The listing builds one solid part. Answer for the finished solid, in the listing's coordinates (mm). A direction names the side the tool comes from. Give positions to 0.01 mm unless a question says otherwise; leave off trailing zeros. Write each loop counter-clockwise with the first axis right and the second up, starting at its lowest first coordinate (ties: lowest second). Pieces come first, ordered by that corner, then holes. Notation, with made-up numbers: (-22, -20.75) - (-2, -20.75) arc R36 ccw to (-2, 18.25) - close; hole circle Ø3 at (-19, 71). An arc over 180 degrees is marked (long way). Answer in a Markdown table with one row per item. Add a question column.
from build123d import *

# Parameters (mm, degrees)
PAD043_DEPTH    = 15
POCKET057_DEPTH = 13
SKETCH118_R     = 1.65
SKETCH118_R_2   = 1.7
SKETCH118_R_3   = 20
POCKET058_DEPTH = 15
POCKET059_DEPTH = 5


with BuildPart() as part:
    # Sketch116 → Pad043 (new body)
    with BuildSketch(Plane.YZ):
        with BuildLine():
            Line((27.5, -9.253658), (27.5, -51.25))
            Line((27.5, -51.25), (-27.5, -51.25))
            Line((-27.5, -51.25), (-27.5, -9.253658))
            ThreePointArc((-20.340323, 1.39583), (-25.543681, -2.837417), (-27.5, -9.253658))
            ThreePointArc((-20.340323, 1.39583), (-18.530459, 2.868264), (-17.85, 5.1))
            ThreePointArc((-12.15, 5.1), (-15, 7.95), (-17.85, 5.1))
            ThreePointArc((-12.15, 5.1), (-11.315254, 3.084746), (-9.3, 2.25))
            Line((-9.3, 2.25), (9.3, 2.25))
            ThreePointArc((9.3, 2.25), (11.315254, 3.084746), (12.15, 5.1))
            ThreePointArc((17.85, 5.1), (15, 7.95), (12.15, 5.1))
            ThreePointArc((17.85, 5.1), (18.530459, 2.868264), (20.340323, 1.39583))
            ThreePointArc((27.5, -9.253658), (25.543681, -2.837417), (20.340323, 1.39583))
        make_face()
    extrude(amount=-PAD043_DEPTH)

    # Sketch117 (on Face14 of Pad043) → Pocket057 (cut)
    with BuildSketch(Plane(origin=(-15, 0, 0), x_dir=(0, -1, 0), z_dir=(-1, 0, 0))):
        with BuildLine():
            Line((-26, -9.253658), (-26, -51.25))
            Line((-26, -51.25), (26, -51.25))
            Line((26, -51.25), (26, -9.253658))
            ThreePointArc((26, -9.253658), (23.071068, -2.18259), (16, 0.746342))
            Line((-16, 0.746342), (16, 0.746342))
            ThreePointArc((-16, 0.746342), (-23.071068, -2.18259), (-26, -9.253658))
        make_face()
    extrude(amount=-POCKET057_DEPTH, mode=Mode.SUBTRACT)

    # Sketch118 (on Face4 of Pocket057) → Pocket058 (cut)
    with BuildSketch(Plane.YZ):
        with Locations((-15, 5.1)):
            Circle(SKETCH118_R)
        with Locations((15, 5.1)):
            Circle(SKETCH118_R)
        with Locations((22.4, -44.05)):
            Circle(SKETCH118_R_2)
        with Locations((-20.9, -5.25)):
            Circle(SKETCH118_R_2)
        with Locations((2, -26.25)):
            Circle(SKETCH118_R_3)
    extrude(amount=-POCKET058_DEPTH, mode=Mode.SUBTRACT)

    # Sketch119 (on Face11 of Pocket058) → Pocket059 (cut)
    with BuildSketch(Plane(origin=(0, -27.5, 0), x_dir=(0, 0, 1), z_dir=(0, -1, 0))):
        Polygon((-51.25, 15), (-28.815971, 15), (-38.35, 7), (-51.25, 7), align=None)
    extrude(amount=-POCKET059_DEPTH, mode=Mode.SUBTRACT)


with BuildPart() as part_1:
    # Body016 placement: moved
    add(part.part.moved(Location((32, 0, 0))))


solid = part_1.part
1. Section C-C (z = -31.5) is taken. Give the vertices of the cut face in (x, y), and give its area (3 significant figures).
2. Section B-B (x = 25.75) is taken. Give the vertices of the cut face in (y, z), and give its area (3 significant figures).
3. Section A-A (y = 2) is taken. Give the vertices of the cut face in (x, z), and give its area (3 significant figures).
4. Given pin 1 Ø4 at (y, z) = (-5, -11) entering from +X; pin 2 Ø4 at (x, y) = (26.5, 13.5) entering from -Z; pin 3 Ø8 at (x, y) = (20, 13.5) entering from -Z; pin 4 Ø1 at (x, z) = (30.5, -3) entering from -Y, each flat-ended and moving along its own axis, determine where each tip first touches the part or whether it passes through.
5. Section D-D (y = -15) is taken. Give the vertices of the cut face in (x, z), and give its area (3 significant figures).
6. A tool of negligible diameter and unlimited length cuts with its end or side. For faces 5 (the face through (20.944, -26.76, -33.516)), 6 (the face through (25, 0, 2.25)), 7 (the face through (23.41, -23.15, -2.26)), 8 (the face through (32, -18, -21)), from which of +Z, -Z, +X, -X, +Y, -Y can it reach the whole face along a straight path? Write none if from no direction.
7. Straight lines are drawn through the part: L1, parallel to Y at x = 18, z = -28.5; L2, parallel to Z at x = 31, y = 2; L3, parallel to Y at x = 26.5, z = 4.5. For each, find the intervals that lie inside material, in ascending order. Write a range as [from, to].
8. The mould has two halves that part along Z. Classify faces 1 (the face through (23, 26, -30)), 2 (the face through (31, -22.6, -5.2)), 3 (the face through (23, 0, 0.746)), 4 (the face through (24.6, 25.6, -2.92)): +Z half, -Z half, draft (parallel to the pull), parting line (faces both ways), or undercut.
Geometry check:
| question | item | result |
|---|---|---|
| 1 | outline | (17, 26) - (30, 26) - (30, 21.3) - (32, 21.3) - (32, 27.5) - (17, 27.5) - close; (19.25, -27.5) - (32, -27.5) - (32, -17.3) - (30, -17.3) - (30, -26) - (19.25, -26) - close |
| 1 | area | 68.4 mm² |
| 2 | outline | (-27.5, -51.25) - (-26, -51.25) - (-26, -9.25) arc R10 cw to (-16, 0.75) - (16, 0.75) arc R10 cw to (26, -9.25) - (26, -51.25) - (27.5, -51.25) - (27.5, -9.25) arc R11.5 ccw to (20.34, 1.4) arc R4 cw to (17.85, 5.1) arc R2.85 ccw to (12.15, 5.1) arc R2.85 cw to (9.3, 2.25) - (-9.3, 2.25) arc R2.85 cw to (-12.15, 5.1) arc R2.85 ccw to (-17.85, 5.1) arc R4 cw to (-20.34, 1.4) arc R11.5 ccw to (-27.5, -9.25) - close; hole circle Ø3.3 at (-15, 5.1); hole circle Ø3.3 at (15, 5.1) |
| 2 | area | 272 mm² |
| 3 | outline | (17, 0.75) - (30, 0.75) - (30, -6.25) - (32, -6.25) - (32, 2.25) - (17, 2.25) - close; (30, -51.25) - (32, -51.25) - (32, -46.25) - (30, -46.25) - close |
| 3 | area | 46.5 mm² |
| 4 | pin 1 | through |
| 4 | pin 2 | z = 0.75 |
| 4 | pin 3 | z = 0.63 |
| 4 | pin 4 | y = -25.96 |
| 5 | outline | (17, 0.75) - (30, 0.75) - (30, -15.71) - (32, -15.71) - (32, 3.45) - (17, 3.45) - close; (17, 6.75) - (32, 6.75) - (32, 7.95) - (17, 7.95) - close; (30, -51.25) - (32, -51.25) - (32, -36.79) - (30, -36.79) - close |
| 5 | area | 120 mm² |
| 6 | face 5 | -Z, -X, -Y |
| 6 | face 6 | +Z, +X, -X |
| 6 | face 7 | -Z, -X |
| 6 | face 8 | +Z, -Z, +X, +Y, -Y |
| 7 | L1 | [-27.5, -26], [26, 27.5] |
| 7 | L2 | [-51.25, -46.25], [-6.25, 2.25] |
| 7 | L3 | [-17.9, -16.54], [-13.46, -12.09], [12.09, 13.46], [16.54, 17.9] |
| 8 | face 1 | draft |
| 8 | face 2 | undercut |
| 8 | face 3 | -Z half |
| 8 | face 4 | +Z half |
